from build123d import *

# Parameters (mm, degrees)
CROQUIS1_W              = 60
CROQUIS1_H              = 60
SALIENTE_EXTRUIR1_DEPTH = 60
CROQUIS2_W              = 30
CROQUIS2_H              = 30
CORTAR_EXTRUIR1_DEPTH   = 30
CORTAR_EXTRUIR2_DEPTH   = 30


with BuildPart() as part:
    # Croquis1 → Saliente-Extruir1 (new body)
    with BuildSketch(Plane(origin=(0, 0, 0), x_dir=(1, 0, 0), z_dir=(0, 1, 0))):
        with Locations((30, -30)):
            Rectangle(CROQUIS1_W, CROQUIS1_H)
    extrude(amount=SALIENTE_EXTRUIR1_DEPTH)

    # Croquis2 → Cortar-Extruir1 (cut)
    with BuildSketch(Plane(origin=(0, 60, 0), x_dir=(1, 0, 0), z_dir=(0, 1, 0))):
        with Locations((45, -45)):
            Rectangle(CROQUIS2_W, CROQUIS2_H)
    extrude(amount=-CORTAR_EXTRUIR1_DEPTH, mode=Mode.SUBTRACT)

    # Croquis3 → Cortar-Extruir2 (cut)
    with BuildSketch(Plane.XY.offset(30)):
        Polygon((30, 60), (60, 30), (60, 60), align=None)
    extrude(amount=-CORTAR_EXTRUIR2_DEPTH, mode=Mode.SUBTRACT)


solid = part.part
Build history of the part. All positions in model axes, mm. A direction names the side the tool comes from. Round coordinates to 2 decimals unless told otherwise and drop trailing zeros. Write each loop counter-clockwise with the first axis right and the second up, starting at its lowest first coordinate (ties: lowest second). Pieces come first, ordered by that corner, then holes. Notation, with made-up numbers: M -34,24 L -2,24 A23 ccw -2,33 Z; hole C -30,19 d9. An arc over 180 degrees is marked long. Answer as a JSON object with one key per item and string values. Group by question number.
(1) Which spindle directions (+Z, -Z, +X, -X, +Y, -Y) get a long thin tool onto all of the face, cutting with end or side? Do faces 1 (the flat face through (38, 39, 30)), 2 (the flat face through (0, 30, 30)). Say none if no direction does.
(2) Cut at A-A (x = 56). Give the cut face in (y, z).
(3) Cut at C-C (z = 11.5). Give the cut face in (x, y).
(4) Flat gauge pins, fed straight in: pin 1 (2 mm diameter, centred on x = 26.5, z = 39.5, fed in from -Y); pin 2 (1.5 mm diameter, centred on x = 31.5, z = 24.5, fed in from +Y); pin 3 (12 mm diameter, centred on x = 51, y = 50.5, fed in from +Z); pin 4 (9 mm diameter, centred on x = 49, z = 50, fed in from +Y). Where does each tip first touch, or does it go through?
(5) Cut at B-B (y = 55). Give the cut face in (x, z).
(6) Drill centre line: L1, parallel to Z at x = 30.5, y = 45. Where is it in solid material? Low to high.
Responses:
{
 "1": {"face 1": "+Z, +X, +Y", "face 2": "+Z, -Z, -X, +Y, -Y"},
 "2": {"outline": "M 0,0 L 34,0 L 34,30 L 30,30 L 30,60 L 0,60 Z"},
 "3": {"outline": "M 0,0 L 60,0 L 60,30 L 30,60 L 0,60 Z"},
 "4": {"pin 1": "stops at y = 0", "pin 2": "stops at y = 59.25", "pin 3": "passes through", "pin 4": "stops at y = 30"},
 "5": {"outline": "M 0,0 L 35,0 L 35,30 L 30,30 L 30,60 L 0,60 Z"},
 "6": {"L1": "z = 0 to 30"}
}
